from build123d import *

# Parameters (mm, degrees)
SKETCH1_W                      = 86.201
SKETCH1_H                      = 71.913
BOSS_EXTRUDE1_DEPTH            = 1.5
FILLET1_R                      = 3
F_2_56_TAPPED_HOLE1_AT_2_COUNT = 2
F_2_56_TAPPED_HOLE1_AT_2_PITCH = 80.201
F_2_56_TAPPED_HOLE1_AT_3_COUNT = 2
F_2_56_TAPPED_HOLE1_AT_3_PITCH = 103.811001199
F_2_56_TAPPED_HOLE1_AT_4_COUNT = 2
F_2_56_TAPPED_HOLE1_AT_4_PITCH = 65.913
CUT_EXTRUDE1_START             = -0.25
CUT_EXTRUDE1_DEPTH             = 0.25


# Read off the part's stored shape, not the designer's step: Cut-Extrude1
with BuildPart() as part:
    # Sketch1 → Boss-Extrude1 (new body)
    with BuildSketch(Plane(origin=(0, 0, 0), x_dir=(1, 0, 0), z_dir=(0, 1, 0))):
        Rectangle(SKETCH1_W, SKETCH1_H)
    extrude(amount=BOSS_EXTRUDE1_DEPTH)

    # Fillet1
    fillet1_edges = [part.edges().sort_by_distance(p)[0] for p in [
        (43.1005, 0.75, 35.9565),
        (-43.1005, 0.75, 35.9565),
        (-43.1005, 0.75, -35.9565),
        (43.1005, 0.75, -35.9565),
    ]]
    fillet(fillet1_edges, radius=FILLET1_R)

    # Sketch4 → #2-56 Tapped Hole1 (revolve, cut)
    with BuildSketch(Plane(origin=(-40.1005, 0, 32.9565), x_dir=(0, 0, -1), z_dir=(1, 0, 0))):
        Polygon((0, 0), (0, 1.5), (0.889, 1.5), (0.889, 0.889), (1.778, 0), align=None)
    f_2_56_tapped_hole1 = revolve(axis=Axis((-40.1005, -6.35, 32.9565), (0, 1, 0)), mode=Mode.SUBTRACT)

    # #2-56 Tapped Hole1 at 2: #2-56 Tapped Hole1 ×2
    with Locations(*[(i * F_2_56_TAPPED_HOLE1_AT_2_PITCH, 0, 0) for i in range(1, F_2_56_TAPPED_HOLE1_AT_2_COUNT)]):
        add(f_2_56_tapped_hole1, mode=Mode.SUBTRACT)

    # #2-56 Tapped Hole1 at 3: #2-56 Tapped Hole1 ×2
    with Locations(*[Vector(0.7725674453907951, 0, -0.634932706924396) * (i * F_2_56_TAPPED_HOLE1_AT_3_PITCH) for i in range(1, F_2_56_TAPPED_HOLE1_AT_3_COUNT)]):
        add(f_2_56_tapped_hole1, mode=Mode.SUBTRACT)

    # #2-56 Tapped Hole1 at 4: #2-56 Tapped Hole1 ×2
    with Locations(*[(0, 0, -i * F_2_56_TAPPED_HOLE1_AT_4_PITCH) for i in range(1, F_2_56_TAPPED_HOLE1_AT_4_COUNT)]):
        add(f_2_56_tapped_hole1, mode=Mode.SUBTRACT)

    # Cut-Extrude1 outline → Cut-Extrude1 (cut)
    with BuildSketch(Plane(origin=(0, 1.5, 0), x_dir=(1, 0, 0), z_dir=(0, 1, 0)).offset(CUT_EXTRUDE1_START)):
        Polygon((-13.990667708, -16.934130724), (-9.929224496, -21.049984667), (9.929227007, -21.049984667), (13.990670219, -16.934130724), align=None)
        Polygon((-18.255824334, 15.410771968), (-9.171914583, 2.791562203), (-0.811527801, 2.791562203), align=None)
        Polygon((18.255804305, 15.410771968), (0.811507772, 2.791562203), (9.171894554, 2.791562203), align=None)
        Polygon((-9.194466068, 10.573407227), (-1.405683839, 4.516178709), (-9.194466068, 21.678326178), align=None)
        Polygon((-13.990667708, -12.320150377), (-9.929224496, -16.436026859), (9.929227007, -16.436026859), (13.990670219, -12.320150377), align=None)
        Polygon((-13.990667708, -7.70619257), (-9.929201956, -11.822069052), (9.929204467, -11.822069052), (13.990670219, -7.70619257), align=None)
        Polygon((-13.990667708, -3.092234762), (-9.929224496, -7.208088705), (9.929227007, -7.208088705), (13.990670219, -3.092234762), align=None)
        Polygon((-13.990667708, 1.521745585), (-9.929224496, -2.594130897), (9.929227007, -2.594130897), (13.990670219, 1.521745585), align=None)
        Polygon((0, 3.801099501), (3.926067099, 12.833705067), (0, 30.78030555), (-3.926067099, 12.833705067), align=None)
        Polygon((1.405683839, 4.516178709), (9.194466068, 10.573407227), (9.194466068, 21.678326178), align=None)
        Polygon((-6.186825635, -29.4565), (6.186825635, -29.4565), (13.990662514, -21.548093926), (-13.990662514, -21.548093926), align=None)
    extrude(amount=CUT_EXTRUDE1_DEPTH, mode=Mode.SUBTRACT)


solid = part.part
The listing builds one solid part. Answer for the finished solid, in the listing's coordinates (mm). A direction names the side the tool comes from. Give positions to 0.01 mm unless a question says otherwise; leave off trailing zeros. Order: outer loops, then holes, each group sorted by start corner. A loop starts at its lowest first (then second) coordinate and runs counter-clockwise, first axis right, second up. Notation, with made-up numbers: (81, 49.25) - (131, 49.25) arc R16 cw to (131, 72.25) - close; hole circle Ø11 at (71, -23.5). An arc over 180 degrees is marked (long way). One line per item, written item: value. Start each with the question number.
1) Given pin 1 Ø2 at (x, z) = (-40.1, 32.96) entering from -Y; pin 2 Ø1.2 at (x, z) = (7, 18.5) entering from +Y, each flat-ended and moving along its own axis, determine where each tip first touches the part or whether it passes through.
2) Find the intervals of material crossed by L1, parallel to Y at x = -1, z = -14; L2, parallel to Z at x = -17.5, y = 1.35, in increasing order.
3) A cutting plane is placed at B-B on z = 9. Give the vertices of the cut face in (x, y).
4) A cutting plane is placed at A-A on z = -6. Give the vertices of the cut face in (x, y), then the cut area to 3 significant figures.
5) A cutting plane is placed at C-C on z = 20. Give the vertices of the cut face in (x, y), then the cut area to 3 significant figures.
6) A tool of negligible diameter and unlimited length cuts with its end or side. For faces 1 (the face through (40.89, 1.19, 32.55)), 2 (the face through (6, 1.25, -13)), from which of +Z, -Z, +X, -X, +Y, -Y can it reach the whole face along a straight path? Write none if from no direction.
Answer sheet:
1. pin 1: stops at y = 0.77
1. pin 2: stops at y = 1.25
2. L1: y = 0 to 1.25
2. L2: z = -35.96 to -14.86, -14.36 to 35.96
3. outline: (-43.1, 0) - (43.1, 0) - (43.1, 1.5) - (12.71, 1.5) - (12.71, 1.25) - (-12.71, 1.25) - (-12.71, 1.5) - (-43.1, 1.5) - close
4. outline: (-43.1, 0) - (43.1, 0) - (43.1, 1.5) - (11.48, 1.5) - (11.48, 1.25) - (5.25, 1.25) - (5.25, 1.5) - (3.31, 1.5) - (3.31, 1.25) - (2.08, 1.25) - (2.08, 1.5) - (0.96, 1.5) - (0.96, 1.25) - (-0.96, 1.25) - (-0.96, 1.5) - (-2.08, 1.5) - (-2.08, 1.25) - (-3.31, 1.25) - (-3.31, 1.5) - (-5.25, 1.5) - (-5.25, 1.25) - (-11.48, 1.25) - (-11.48, 1.5) - (-43.1, 1.5) - close
4. area: 125 mm2
5. outline: (-43.1, 0) - (43.1, 0) - (43.1, 1.5) - (10.97, 1.5) - (10.97, 1.25) - (-10.97, 1.25) - (-10.97, 1.5) - (-43.1, 1.5) - close
5. area: 124 mm2
6. face 1: +Y, -Y
6. face 2: +Y
